```python
from build123d import *

# Parameters (mm, degrees)
SKETCH1_R                   = 10
SMALLRING_DEPTH             = 13
SKETCH4_R                   = 19
SKETCH4_R_2                 = 2
BIGRING_DEPTH               = 5
M4_TAPPED_HOLE1_D           = 3.3
M4_TAPPED_HOLE1_DEPTH       = 10.1
M4_TAPPED_HOLE1_CSINK_D     = 4.05
M4_TAPPED_HOLE1_CSINK_ANGLE = 90
M4_TAPPED_HOLE1_TIP         = 0.991420021
SKETCH42_R                  = 5
MOTOR_SHAFT_HOLE_DEPTH      = 20
SKETCH43_W                  = 3
SKETCH43_H                  = 4
KEYWAY_DEPTH                = 18


with BuildPart() as part:
    # Sketch1 → SmallRing (new body)
    with BuildSketch(Plane(origin=(0, 0, 0), x_dir=(0, 0, -1), z_dir=(1, 0, 0))):
        Circle(SKETCH1_R)
    extrude(amount=SMALLRING_DEPTH)

    # Sketch4 → BigRing (add)
    with BuildSketch(Plane.ZY):
        Circle(SKETCH4_R)
        with Locations((-10.606601718, 10.606601718)):
            Circle(SKETCH4_R_2, mode=Mode.SUBTRACT)
        with Locations((10.606601718, 10.606601718)):
            Circle(SKETCH4_R_2, mode=Mode.SUBTRACT)
        with Locations((10.606601718, -10.606601718)):
            Circle(SKETCH4_R_2, mode=Mode.SUBTRACT)
        with Locations((-10.606601718, -10.606601718)):
            Circle(SKETCH4_R_2, mode=Mode.SUBTRACT)
    extrude(amount=BIGRING_DEPTH)

    # M4 Tapped Hole1
    with Locations(Plane(origin=(8, 10, 0), x_dir=(1, 0, 0), z_dir=(0, 1, 0))):
        with Locations((0, 0)):
            CounterSinkHole(M4_TAPPED_HOLE1_D / 2, M4_TAPPED_HOLE1_CSINK_D / 2, depth=M4_TAPPED_HOLE1_DEPTH, counter_sink_angle=M4_TAPPED_HOLE1_CSINK_ANGLE)
            with Locations((0, 0, -(M4_TAPPED_HOLE1_DEPTH + M4_TAPPED_HOLE1_TIP / 2))):  # 118° drill point
                Cone(0, M4_TAPPED_HOLE1_D / 2, M4_TAPPED_HOLE1_TIP, mode=Mode.SUBTRACT)

    # Sketch42 → Motor Shaft Hole (cut)
    with BuildSketch(Plane(origin=(13, 0, 0), x_dir=(0, 0, -1), z_dir=(1, 0, 0))):
        Circle(SKETCH42_R)
    extrude(amount=-MOTOR_SHAFT_HOLE_DEPTH, mode=Mode.SUBTRACT)

    # Sketch43 → Keyway (cut)
    with BuildSketch(Plane(origin=(13, 0, 0), x_dir=(0, 0, -1), z_dir=(1, 0, 0))):
        with Locations((0, 5)):
            Rectangle(SKETCH43_W, SKETCH43_H)
    extrude(amount=-KEYWAY_DEPTH, mode=Mode.SUBTRACT)


solid = part.part
```
CAD build for the part. Positions are in the model's coordinates, mm. A direction names the side the tool comes from. Coordinates: 2 decimals unless noted, no trailing zeros. Order: outer loops, then holes, each group sorted by start corner. A loop starts at its lowest first (then second) coordinate and runs counter-clockwise, first axis right, second up.
(1) Drill centre lines: L1, parallel to Y at x = 1.75, z = 0; L2, parallel to X at y = -15.5, z = 5.5; L3, parallel to Z at x = -3.5, y = 4. Where is each one in solid material? Low to high.
Solution:
L1: y = -10 to -5, 7 to 10
L2: x = -5 to 0
L3: z = -18.57 to -3, 3 to 18.57
(2) Saw through at A-A, the plane z = 0. Write the cut outline in (x, y) (3 decimals).
Solution:
outline: (-5, -19) - (0, -19) - (0, -10) - (13, -10) - (13, -5) - (-5, -5) - close; (-5, 7) - (6.35, 7) - (6.35, 9.625) - (5.975, 10) - (0, 10) - (0, 19) - (-5, 19) - close; (9.65, 7) - (13, 7) - (13, 10) - (10.025, 10) - (9.65, 9.625) - close
(3) Saw through at D-D, the plane y = -9.5. Write the cut outline in (x, z), and give its area (3 significant figures).
Solution:
outline: (-5, -16.45) - (0, -16.45) - (0, -12.27) - (-5, -12.27) - close; (-5, -8.94) - (0, -8.94) - (0, -3.12) - (13, -3.12) - (13, 3.12) - (0, 3.12) - (0, 8.94) - (-5, 8.94) - close; (-5, 12.27) - (0, 12.27) - (0, 16.45) - (-5, 16.45) - close
area: 212 mm2
(4) Mould opens along Z. For faces 5 (the face through (11, 6, -1.5)), 6 (the face through (-5, -4, 4)), 7 (the face through (-2.465, -16.856, 8.767)) say: released by +Z, released by -Z, zero draft, split by the parting line, or undercut.
Solution:
face 5: undercut
face 6: zero draft
face 7: split by the parting line
(5) Saw through at B-B, the plane y = 0. Write the cut outline in (x, z).
Solution:
outline: (-5, -19) - (0, -19) - (0, -10) - (13, -10) - (13, -5) - (-5, -5) - close; (-5, 5) - (13, 5) - (13, 10) - (0, 10) - (0, 19) - (-5, 19) - close
(6) Which spindle directions (+Z, -Z, +X, -X, +Y, -Y) get a long thin tool onto all of the face, cutting with end or side? Do faces 1 (the face through (1, 6, 1.5)), 2 (the face through (13, -2, 5)), 3 (the face through (9.65, 7.68, -0.07)), 4 (the face through (6.41, -9.76, 2.17)). Say none if no direction does.
Solution:
face 1: +X, -X
face 2: +Z, -Z, +X, +Y, -Y
face 3: +Y
face 4: +X
(7) Pin check, flat tips, straight feed: pin 1 Ø5 at (x, z) = (9.5, 6) entering from -Y; pin 2 Ø3 at (x, z) = (-1.5, 15) entering from +Y; pin 3 Ø2.5 at (x, y) = (-0.5, 6) entering from -Z; pin 4 Ø3 at (y, z) = (10.61, 10.61) entering from -X. Stop position of each tip, or through.
Solution:
pin 1: stops at y = -9.37
pin 2: stops at y = 13.37
pin 3: stops at z = -18.4
pin 4: passes through
(8) Saw through at C-C, the plane x = 2.75. Write the cut outline in (y, z).
Solution:
outline: circle Ø20 at (0, 0); hole (4.77, -1.5) - (7, -1.5) - (7, 1.5) - (4.77, 1.5) arc R5 ccw (long way) to start
